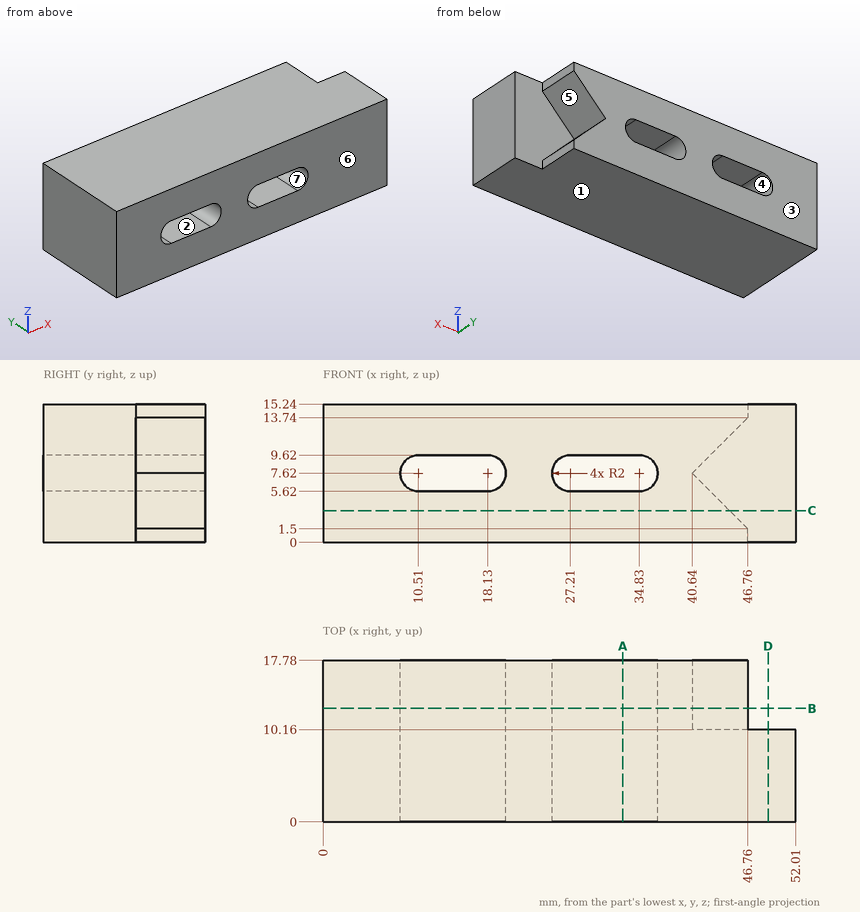
Study the drawing (mm; zero at the part's minimum x, y, z) and answer. A direction names the side the tool comes from. Give positions to 0.01 mm unless a question says otherwise; leave off trailing zeros. Loops run counter-clockwise (first coordinate to the right, second up) from the corner with the lowest first, then second, coordinate; pieces in that order, holes last. Notation, with made-up numbers: (12.25, 12.25) -> (28.25, 12.25) arc R21 cw to (28.25, 19.25) -> close; hole circle Ø11 at (-39, 53.25). An arc over 180 degrees is marked (long way). Use a Markdown table: item, result. Add a question column.
1) The part is cut by section A-A, the plane x = 33. Determine the outline of the cut face in (y, z), plus the area to 3 significant figures.
2) Consider line 1 along X through (y, z) = (5, 8); line 2 along Z through (x, y) = (14.5, 3.5); line 3 along X through (y, z) = (3.75, 8.75). Determine where each line is inside the solid, lowest interval first.
3) The part is cut by section C-C, the plane z = 3.5. Determine the outline of the cut face in (x, y), plus the area to 3 significant figures.
4) The part is cut by section D-D, the plane x = 49. Determine the outline of the cut face in (y, z), plus the area to 3 significant figures.
5) This flat-tipped pin is pushed along its axis until it touches: P1, Ø0.8, axis at y = 13.5, z = 15, coming from the +X side. Where does it stop, or does it pass through?
6) The part is cut by section B-B, the plane y = 12.5. Determine the outline of the cut face in (x, z).
7) For a pull along Z with two mould halves and no side action, classify the marked faces 1, 2, 3 and 4 as +Z half, -Z half, draft (parallel to the pull), parting line (faces both ways), or undercut.
8) Which of the six approach directions +Z, -Z, +X, -X, +Y, -Y give full straight-line access (tool end or side, diameter ignored) to the marked faces 5, 6 and 7?
Reported:
| question | item | result |
|---|---|---|
| 1 | outline | (0, 0) -> (17.78, 0) -> (17.78, 5.62) -> (0, 5.62) -> close; (0, 9.62) -> (17.78, 9.62) -> (17.78, 15.24) -> (0, 15.24) -> close |
| 1 | area | 200 mm^2 |
| 2 | line 1 | x = 0 to 8.55, 20.09 to 25.25, 36.79 to 52.01 |
| 2 | line 2 | z = 0 to 5.62, 9.62 to 15.24 |
| 2 | line 3 | x = 0 to 8.86, 19.78 to 25.56, 36.48 to 52.01 |
| 3 | outline | (0, 0) -> (52.01, 0) -> (52.01, 10.16) -> (44.76, 10.16) -> (44.76, 17.78) -> (0, 17.78) -> close |
| 3 | area | 869 mm^2 |
| 4 | outline | (0, 0) -> (10.16, 0) -> (10.16, 15.24) -> (0, 15.24) -> close |
| 4 | area | 155 mm^2 |
| 5 | P1 | stops at x = 46.76 |
| 6 | outline | (0, 0) -> (46.76, 0) -> (46.76, 1.5) -> (40.64, 7.62) -> (46.76, 13.74) -> (46.76, 15.24) -> (0, 15.24) -> close; hole (10.51, 5.62) -> (18.13, 5.62) arc R2 ccw to (18.13, 9.62) -> (10.51, 9.62) arc R2 ccw to start; hole (27.21, 5.62) -> (34.83, 5.62) arc R2 ccw to (34.83, 9.62) -> (27.21, 9.62) arc R2 ccw to start |
| 7 | face 1 | -Z half |
| 7 | face 2 | undercut |
| 7 | face 3 | draft |
| 7 | face 4 | undercut |
| 8 | face 5 | +X, +Y |
| 8 | face 6 | +Z, -Z, +X, -X, -Y |
| 8 | face 7 | +Y, -Y |
